Input: part model. Units: mm. Frame: model coordinates. Face numbers are marked on the shaded views. A direction names the side the tool comes from. Coordinates: 2 decimals unless noted, no trailing zeros. Order: outer loops, then holes, each group sorted by start corner. A loop starts at its lowest first (then second) coordinate and runs counter-clockwise, first axis right, second up. Notation, with made-up numbers: (37, 1) - (47, 1) arc R28 ccw to (47, 35) - close; hole circle Ø2 at (-37, 25.25). An arc over 180 degrees is marked (long way). Answer as CSV lines item,"result". Start each with the question number.
Item 1: Section C-C (y = 4). Output: boundary loops of the cut face in (x, z), and give its area (3 significant figures).
Item 2: Draft query along Z for the marked faces 1, 2 and 3. Return one class per face: +Z half, -Z half, draft (parallel to the pull), parting line (faces both ways), or undercut.
Item 3: First-contact query: pin 1 (4 mm diameter, centred on x = 38.5, z = 40, fed in from +Y); pin 2 (1 mm diameter, centred on x = 37, y = 3.5, fed in from -Z); pin 3 (0.8 mm diameter, centred on x = 2.5, z = 20, fed in from +Y); pin 4 (4 mm diameter, centred on x = 3.54, z = 25.08, fed in from +Y) (3 decimals). Flat tips, straight axial feed; report the tip coordinate or a pass-through.
Item 4: Access query for the marked faces 4, 5, 6 and 7. Directions: +Z, -Z, +X, -X, +Y, -Y. A direction counts if a zero-diameter tool reaches every point of the face in a straight line with its end or side. Return the directions, or none.
Item 5: Material intervals for line 1 along X through (y, z) = (2.5, 25.08); line 2 along Z through (x, y) = (3.54, 2.5); line 3 along Z through (x, y) = (38.5, 3.9), sorted ascending.
Item 6: Section B-B (z = 14.92). Output: boundary loops of the cut face in (x, y).
Item 7: Section A-A (x = 0). Output: boundary loops of the cut face in (y, z), and give its area (3 significant figures).
Item 8: Section D-D (z = 30). Output: boundary loops of the cut face in (x, y), and give its area (3 significant figures).
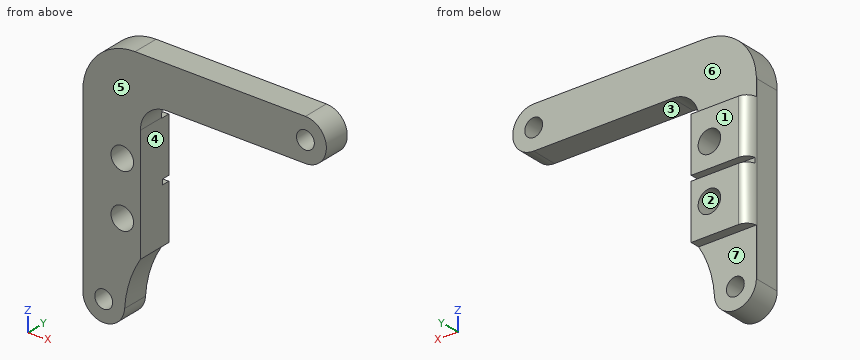
from build123d import *

# Parameters (mm, degrees)
BOSS_EXTRU_1_DEPTH      = 5
D_GAGEMENT_M31_D        = 3.4
ESQUISSE5_W             = 11
ESQUISSE5_H             = 21.78
BOSS_EXTRU_2_DEPTH      = 1.78
ESQUISSE6_W             = 1
ESQUISSE6_H             = 1.55
ENL_V_MAT_EXTRU_1_DEPTH = 65.375604075
D_GAGEMENT_M42_D        = 4.3
ESQUISSE9_W             = 5.11
ESQUISSE9_H             = 5
BOSS_EXTRU_3_DEPTH      = 3
CONG_2_R                = 5
CONG_3_R                = 10
CONG_4_R                = 2
CONG_5_R                = 20


with BuildPart() as part:
    # Esquisse2 → Boss.-Extru.1 (new body)
    with BuildSketch(Plane(origin=(0, 0, 0), x_dir=(1, 0, 0), z_dir=(0, 1, 0))):
        with BuildLine():
            Line((4, -36), (38.5, -36))
            ThreePointArc((38.5, -36), (42.5, -40), (38.5, -44))
            Line((38.5, -44), (-4, -44))
            Line((-4, -44), (-4, 0))
            ThreePointArc((-4, 0), (0, 4), (4, 0))
            Line((4, 0), (4, -9.11))
            Line((4, -9.11), (7, -9.11))
            Line((7, -9.11), (7, -30.89))
            Line((7, -30.89), (4, -30.89))
            Line((4, -30.89), (4, -36))
        make_face()
    extrude(amount=BOSS_EXTRU_1_DEPTH)

    # Dégagement M31 (through all)
    with Locations(Plane(origin=(0, 5, 0), x_dir=(1, 0, 0), z_dir=(0, 1, 0))):
        with Locations((0, 0), (38.5, -40)):
            Hole(D_GAGEMENT_M31_D / 2)

    # Esquisse5 → Boss.-Extru.2 (add)
    with BuildSketch(Plane(origin=(0, 5, 0), x_dir=(1, 0, 0), z_dir=(0, 1, 0))):
        with Locations((1.5, -20)):
            Rectangle(ESQUISSE5_W, ESQUISSE5_H)
    extrude(amount=BOSS_EXTRU_2_DEPTH)

    # Esquisse6 → Enlèv. mat.-Extru.1 (cut, through all)
    with BuildSketch(Plane.ZY.offset(4)):
        with Locations((20, 6.005)):
            Rectangle(ESQUISSE6_W, ESQUISSE6_H)
    extrude(amount=-ENL_V_MAT_EXTRU_1_DEPTH, mode=Mode.SUBTRACT)

    # Dégagement M42 (through all)
    with Locations(Plane(origin=(0, 6.78, 0), x_dir=(1, 0, 0), z_dir=(0, 1, 0))):
        with Locations((3.54, -25.08), (3.54, -14.92)):
            Hole(D_GAGEMENT_M42_D / 2)

    # Esquisse9 → Boss.-Extru.3 (add)
    with BuildSketch(Plane(origin=(4, 0, 0), x_dir=(0, 0, -1), z_dir=(1, 0, 0))):
        with Locations((-33.445, 2.5)):
            Rectangle(ESQUISSE9_W, ESQUISSE9_H)
    extrude(amount=BOSS_EXTRU_3_DEPTH)

    # Congé2
    cong_2_edges = [part.edges().sort_by_distance(p)[0] for p in [
        (7, 2.5, 36),
    ]]
    fillet(cong_2_edges, radius=CONG_2_R)

    # Congé3
    cong_3_edges = [part.edges().sort_by_distance(p)[0] for p in [
        (-4, 2.5, 44),
    ]]
    fillet(cong_3_edges, radius=CONG_3_R)

    # Congé4
    # the kernel refuses this fillet: 2 mm, written as the material it takes off along each edge
    with BuildSketch(Plane(origin=(-4, 6.78, -2.89), x_dir=(0, -1, 0), z_dir=(0, 0, 1)), Plane(origin=(-4, 6.78, 8.5), x_dir=(0, -1, 0), z_dir=(0, 0, 1))) as cong_4_piece_1:
        with BuildLine():
            CenterArc((CONG_4_R, CONG_4_R), CONG_4_R, 180, 90)
            Line((0, CONG_4_R), (-CONG_4_R * 0.02, CONG_4_R))
            Line((-CONG_4_R * 0.02, CONG_4_R), (-CONG_4_R * 0.02, -CONG_4_R * 0.02))
            Line((-CONG_4_R * 0.02, -CONG_4_R * 0.02), (CONG_4_R, -CONG_4_R * 0.02))
            Line((CONG_4_R, -CONG_4_R * 0.02), (CONG_4_R, 0))
        make_face()
    extrude(amount=34.39, mode=Mode.SUBTRACT)

    # Congé5
    # the kernel refuses this fillet: 20 mm, written as the material it adds along each edge
    with BuildSketch(Plane(origin=(4, 0, 9.11), x_dir=(1, 0, 0), z_dir=(0, 1, 0))) as cong_5_piece_1:
        with BuildLine():
            CenterArc((19.95301022, 10.611100059), CONG_5_R, 183.585953045, 28.45700877)
            Line((-0.00783163, 9.360183343), (-2.003915815, 9.235091672))
            ThreePointArc((-2.003915815, 9.235091672), (-2, 9.11), (-2, 0))
            Line((-2, 0), (0, -2))
            ThreePointArc((0, -2), (1.5, -2), (1.304698978, -1.061110006))
            Line((1.304698978, -1.061110006), (3, 0))
        make_face()
    extrude(amount=5)


solid = part.part
Determined:
1,outline,"(-4, 0) arc R4 ccw to (3.99, -0.25) arc R20 cw to (7, 9.11) - (7, 31) arc R5 cw to (12, 36) - (38.5, 36) arc R4 ccw to (38.5, 44) - (6, 44) arc R10 ccw to (-4, 34) - close; hole circle Ø3.4 at (0, 0); hole circle Ø4.3 at (3.54, 14.92); hole circle Ø4.3 at (3.54, 25.08); hole circle Ø3.4 at (38.5, 40)"
1,area,"706 mm^2"
2,face 1,"draft"
2,face 2,"undercut"
2,face 3,"-Z half"
3,pin 1,"stops at y = 5"
3,pin 2,"stops at z = 36"
3,pin 3,"stops at y = 5.23"
3,pin 4,"passes through"
4,face 4,"-Z, +X, +Y, -Y"
4,face 5,"+Z, -Z, +X, -X, -Y"
4,face 6,"+Z, +X, -X, +Y"
4,face 7,"-Z, +X, -X, +Y"
5,line 1,"x = -4 to 1.39, 5.69 to 7"
5,line 2,"z = -1.86 to 12.77, 17.07 to 22.93, 27.23 to 43.69"
5,line 3,"z = 36 to 38.3, 41.7 to 44"
6,outline,"(-4, 0) - (1.39, 0) - (1.39, 6.78) - (-2, 6.78) arc R2 ccw to (-4, 4.78) - close; (5.69, 0) - (7, 0) - (7, 6.78) - (5.69, 6.78) - close"
7,outline,"(0, -4) - (5, -4) - (5, -1.7) - (0, -1.7) - close; (0, 1.7) - (5, 1.7) - (5, 9.11) - (6.78, 9.11) - (6.78, 19.5) - (5.23, 19.5) - (5.23, 20.5) - (6.78, 20.5) - (6.78, 30.89) - (5, 30.89) - (5, 42) - (0, 42) - close"
7,area,"250 mm^2"
8,outline,"(-4, 0) - (7, 0) - (7, 6.78) - (-2, 6.78) arc R2 ccw to (-4, 4.78) - close"
8,area,"73.7 mm^2"
